Design review of the part built by this model. Coordinates are the model's own, in mm. A direction names the side the tool comes from. Round coordinates to 2 decimals unless told otherwise and drop trailing zeros. Use a Markdown table: item, result.
Solid Edge part; units mm, degrees
sketch "Sketch1" plane through (0, 0, 0) normal (0, -1, 0) x (1, 0, 0)
  line L0 (-39.5566, 0) -> (62.4434, 0)
  line L1 (50.4434, -60) -> (62.4434, 0)
  line L2 (50.4434, -60) -> (44.4434, -90)
  line L3 (38.4434, -90) -> (44.4434, -90)
  line L4 (38.4434, -90) -> (14.4434, -90)
  line L5 (14.4434, -90) -> (-39.5566, 0)
extrude "Protrusion1" add sketch "Sketch1" along normal mid plane 12
chamfer "Chamfer_1" distance 6 angle 45 2 edges at (-12.5566, 6, -45) (-12.5566, -6, -45)
chamfer "Chamfer_2" distance 6 angle 45 2 edges at (53.4434, 6, -45) (53.4434, -6, -45)
chamfer "Chamfer_3" distance 6 angle 45 2 edges at (29.8825, 6, -90) (29.8825, -6, -90)
sketch "Sketch2" plane through (11.4434, 0, 0) normal (0, 0, 1) x (1, 0, 0)
  line L0 (33.817, 2.9533) -> (38.817, -0.0467)
  line L1 (38.817, -0.0467) -> (33.817, -3.0467)
  line L2 (33.817, 2.9533) -> (33.817, -3.0467)
extrude "ExtrudedCutout_3" cut sketch "Sketch2" against normal blind 2.5
sketch "Sketch3" plane through (47.7603, -0.0467, -2.5) normal (0, 0, 1) x (0.8575, 0.5145, 0)
  circle A0 centre (0.0237, 0.0403) radius 1.25
extrude "ExtrudedCutout_4" cut sketch "Sketch3" against normal blind 2.5
1. Insertion check: pin 1 (2 mm diameter, centred on y = 1.5, z = -0.5, fed in from +X); pin 2 (0.8 mm diameter, centred on x = 48, y = -0.5, fed in from +Z); pin 3 (2 mm diameter, centred on y = 0, z = -22, fed in from -X). Each pin has a flat end and moves straight along its axis. Give the tip position at first contact, or say it passes through.
Check values:
| item | result |
|---|---|
| pin 1 | stops at x = 61.85 |
| pin 2 | stops at z = -5 |
| pin 3 | stops at x = -26.96 |
2. Wall thickness on line 1 along X through (y, z) = (0, -42); line 2 along Z through (x, y) = (2, 5.75); line 3 along X through (y, z) = (-1.5, -47): over which ranges is each line inside the solid? List them lowest first. Write a range as from..to.
Check values:
| item | result |
|---|---|
| line 1 | x = -14.36..54.04 |
| line 2 | z = -58.09..0 |
| line 3 | x = -9.61..51.51 |
3. The part is to be moulded in two halves that separate along X. For faces 1 (the face through (29, 3, -87)), 2 (the face through (-9.6, -3, -44.1)), 3 (the face through (48.825, -0.654, -3.732)), say which applies: pulls with the +X half, pulls with the -X half, needs draft (parallel to the pull), parting line crosses it, or undercut.
Check values:
| item | result |
|---|---|
| face 1 | needs draft |
| face 2 | pulls with the -X half |
| face 3 | undercut |
4. Machinability: for faces 4 (the face through (-9.6, 3, -44.1)), 5 (the face through (47.795, -1.526, -1.232)), which of the approach directions +Z, -Z, +X, -X, +Y, -Y give a long, thin tool a straight path to every point of the face, cutting with its end or side? Answer none if there is none.
Check values:
| item | result |
|---|---|
| face 4 | -Z, -X, +Y |
| face 5 | +Z |
